Autodesk Inventor part; units mm, degrees
ref_plane "Work Plane1" through (0, 0, 110) normal (0, 0, 1) x (1, 0, 0)
ref_plane "Work Plane2" through (-77.5, 605, 280) normal (0, 1, 0) x (1, 0, 0)
ref_plane "Work Plane4" through (0, 0, 110) normal (0, 0, 1) x (1, 0, 0)
sketch "Sketch1" plane through (0, 0, 0) normal (0, 0, 1) x (1, 0, 0)
  line L0 (0, 450) -> (0, 610) construction
  line L1 (-77.5, 610) -> (-77.5, 443.2762)
  line L2 (77.5, 610) -> (77.5, 443.2762)
  arc A0 (77.5, 443.2762) -> (-77.5, 443.2762) centre (0, 0) ccw
  line L3 (-77.5, 610) -> (-77.5, 625)
  line L4 (-77.5, 625) -> (77.5, 625)
  line L5 (77.5, 625) -> (77.5, 610)
  dimension "d7" = 15
extrude "Extrusion1" add sketch "Sketch1" along normal blind 220
sketch "Sketch2" plane through (0, 0, 220) normal (0, 0, 1) x (1, 0, 0)
  arc A0 (77.5, 443.2762) -> (-77.5, 443.2762) centre (0, 0) ccw
  line L0 (77.5, 443.2762) -> (77.5, 625)
  line L1 (77.5, 458.4962) -> (77.5, 625)
  line L2 (77.5, 625) -> (-77.5, 625)
  line L3 (-77.5, 625) -> (-77.5, 458.4962)
  arc A1 (77.5, 458.4962) -> (-77.5012, 458.496) centre (0, 0) ccw
  dimension "d12" = 465
extrude "Extrusion2" add sketch "Sketch2" along normal blind 10
sketch "Sketch3" plane through (0, 0, 230) normal (0, 0, 1) x (1, 0, 0)
  arc A0 (77.5, 443.2762) -> (-77.5, 443.2762) centre (0, 0) ccw
  arc A1 (77.5, 443.2762) -> (-77.5, 443.2762) centre (0, 0) ccw
  line L0 (-77.5, 625) -> (-77.5, 443.2762)
  line L1 (-77.5, 443.2762) -> (-77.5, 625)
  line L2 (-77.5, 625) -> (77.5, 625)
  line L3 (77.5, 625) -> (77.5, 443.2762)
extrude "Extrusion3" add sketch "Sketch3" along normal blind 50
ref_plane "Work Plane1" through (0, 0, 110) normal (0, 0, 1) x (1, 0, 0)
mirror "Mirror1" about plane through (0, 0, 110) normal (0, 0, 1) of "Extrusion2", "Extrusion3"
ref_plane "Work Plane2" through (-77.5, 605, 280) normal (0, 1, 0) x (1, 0, 0)
sketch "Sketch4" plane through (-77.5, 605, 280) normal (0, 1, 0) x (1, 0, 0)
  line L0 (5, 15) -> (5, 325)
  line L1 (150, 15) -> (150, 325)
  line L2 (155, 340) -> (155, 0)
  line L3 (150, 15) -> (5, 15)
  line L4 (150, 325) -> (5, 325)
  point P0 (77.5, 280)
extrude "Extrusion4" cut sketch "Sketch4" against normal up to next
sketch "Sketch5" plane through (77.5, 443.2762, 220) normal (1, 0, 0) x (0, 0, -1)
  line L0 (280, 181.7238) -> (-60, 181.7238)
  line L1 (-60, 181.7238) -> (280, 181.7238)
  line L2 (-10, 0) -> (-60, 0)
  line L3 (-60, 0) -> (-60, 181.7238)
  line L4 (230, 0) -> (280, 0)
  line L5 (280, 181.7238) -> (280, 0)
  line L6 (280, 0) -> (280, 181.7238)
  line L7 (230, 0) -> (280, 0)
  line L8 (220, 15.22) -> (230, 15.22)
  line L9 (230, 0) -> (230, 15.22)
  line L10 (230, 15.22) -> (220, 15.22)
  line L11 (220, 15.22) -> (220, 0)
  line L12 (0, 16.0372) -> (0, 15.22)
  line L13 (0, 0) -> (0, 15.22)
  line L14 (0, 15.22) -> (-10, 15.22)
  line L15 (0, 15.22) -> (-10, 15.22)
  line L16 (-10, 15.22) -> (-10, 0)
  line L17 (-60, 0) -> (-10, 0)
  line L18 (0, 0) -> (220, 0)
  point P0 (220, -443.2762)
extrude "Extrusion5" add sketch "Sketch5" along normal blind 10
mirror "Mirror2" about plane through (0, 0, 0) normal (1, 0, 0) of "Extrusion5"
ref_plane "Work Plane4" through (0, 0, 110) normal (0, 0, 1) x (1, 0, 0)
sketch "Sketch7" plane through (0, 0, 110) normal (0, 0, 1) x (1, 0, 0)
  line L0 (87.5, 625) -> (87.5, 443.2762)
  arc A0 (-87.5, 625) -> (87.5, 625) centre (0, 0) ccw
  arc A1 (-87.5, 517.657) -> (87.5, 517.657) centre (0, 0) ccw
  line L1 (87.5, 517.657) -> (87.5, 625)
  line L2 (-87.5, 625) -> (-87.5, 517.657)
  dimension "d20" = 1050
extrude "Extrusion6" add sketch "Sketch7" along normal mid plane 100
sketch "Sketch8" plane through (0, 0, 160) normal (0, 0, 1) x (1, 0, 0)
  line L0 (0, 0) -> (-251.6368, -373.0669) construction
  line L1 (0, 0) -> (0, -450) construction
  line L2 (0, 0) -> (251.6368, -373.0669) construction
  line L3 (0, 0) -> (0, -450) construction
  line L4 (257.2287, -381.3573) -> (293.5763, -435.2447)
  arc A0 (-87.5, 517.657) -> (87.5, 517.657) centre (0, 0) ccw
  line L5 (-257.2287, -381.3573) -> (-293.5763, -435.2447)
  arc A1 (-293.5763, -435.2447) -> (293.5763, -435.2447) centre (0, 0) ccw
  arc A2 (0, -460) -> (257.2287, -381.3573) centre (0, 0) ccw
  arc A3 (-257.2287, -381.3573) -> (0, -460) centre (0, 0) ccw
  dimension "d24" = 34
  dimension "d25" = 34
  dimension "d28" = 450
  dimension "d29" = 460
extrude "Extrusion7" add sketch "Sketch8" against normal blind 100
sketch "Sketch9" plane through (0, 0, 110) normal (0, 0, 1) x (1, 0, 0)
  arc A0 (293.5763, -435.2447) -> (87.5, 517.657) centre (0, 0) ccw
  arc A1 (507.1111, -135.88) -> (507.1111, 135.88) centre (0, 0) ccw
  line L0 (0, 0) -> (507.1111, 135.88) construction
  line L1 (0, 0) -> (525, 0) construction
  line L2 (0, 0) -> (507.1111, -135.88) construction
  arc A2 (434.6666, -116.4686) -> (434.6666, 116.4686) centre (0, 0) ccw
  line L3 (0, 0) -> (434.6666, 116.4686) construction
  line L4 (0, 0) -> (450, 0) construction
  line L5 (0, 0) -> (434.6666, -116.4686) construction
  line L6 (434.6666, 116.4686) -> (507.1111, 135.88)
  line L7 (507.1111, -135.88) -> (434.6666, -116.4686)
  dimension "d30" = 15
  dimension "d31" = 30
  dimension "d32" = 450
  dimension "d33" = 15
  dimension "d34" = 30
extrude "Extrusion8" add sketch "Sketch9" along normal mid plane 220
sketch "Sketch10" plane through (0, 0, 220) normal (0, 0, 1) x (1, 0, 0)
  line L0 (507.1111, 135.88) -> (434.6666, 116.4686)
  arc A0 (449.1555, -120.3509) -> (449.1555, 120.3509) centre (0, 0) ccw
  arc A1 (507.1111, -135.88) -> (507.1111, 135.88) centre (0, 0) ccw
  arc A2 (507.1111, -135.88) -> (507.1111, 135.88) centre (0, 0) ccw
  line L1 (449.1555, 120.3509) -> (507.1111, 135.88)
  line L2 (507.1111, -135.88) -> (449.1555, -120.3509)
  dimension "d37" = 465
extrude "Extrusion9" add sketch "Sketch10" along normal blind 10
sketch "Sketch11" plane through (0, 0, 230) normal (0, 0, 1) x (1, 0, 0)
  arc A0 (434.6666, -116.4686) -> (434.6666, 116.4686) centre (0, 0) ccw
  line L0 (434.6666, 116.4686) -> (507.1111, 135.88)
  arc A1 (434.6666, -116.4686) -> (434.6666, 116.4686) centre (0, 0) ccw
  arc A2 (507.1111, -135.88) -> (507.1111, 135.88) centre (0, 0) ccw
  arc A3 (507.1111, -135.88) -> (507.1111, 135.88) centre (0, 0) ccw
  line L1 (507.1111, 135.88) -> (434.6666, 116.4686)
  line L2 (507.1111, -135.88) -> (434.6666, -116.4686)
  line L3 (507.1111, -135.88) -> (434.6666, -116.4686)
extrude "Extrusion10" add sketch "Sketch11" along normal blind 30
mirror "Mirror3" about plane through (0, 0, 110) normal (0, 0, 1) of "Extrusion9", "Extrusion10"
mirror "Mirror4" about plane through (0, 0, 0) normal (1, 0, 0) of "Extrusion8", "Extrusion9", "Extrusion10", "Mirror3"
ref_plane "Work Plane3" through (0, 0, 0) normal (1, 0, 0) x (0, 1, 0)
properties part number "source holder"
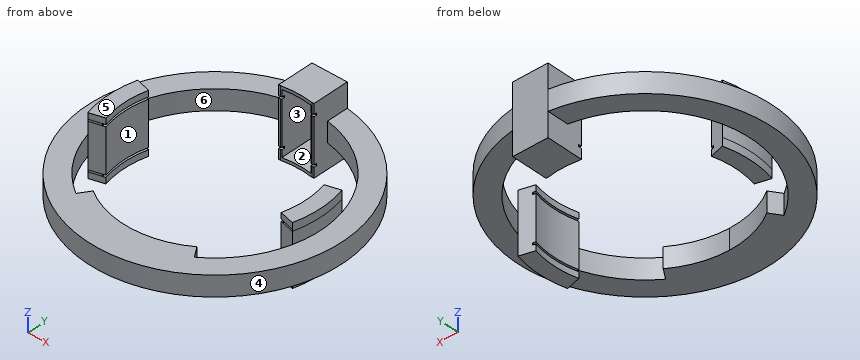
Input: part model. Units: mm. Frame: model coordinates. Face numbers are marked on the shaded views. A direction names the side the tool comes from. Give positions to 0.01 mm unless a question says otherwise; leave off trailing zeros. Loops run counter-clockwise (first coordinate to the right, second up) from the corner with the lowest first, then second, coordinate; pieces in that order, holes last. Notation, with made-up numbers: (-36, 69) - (-10, 69) arc R11 cw to (-10, 76) - close; hole circle Ø7 at (32, 35). An arc over 180 degrees is marked (long way). Use CSV: the item, a comma, the result in double quotes. Start each with the question number.
Item 1: Line query: line 1 (Z direction, x = -2, y = 569.5); line 2 (X direction, y = 501.5, z = 44); line 3 (X direction, y = -399, z = 116). Output: solid intervals per line, ascending.
Item 2: Reachability of the marked faces 1, 2 and 3 from +Z, -Z, +X, -X, +Y, -Y: full face, straight path, thin tool, end or side. Return the list, or none.
Item 3: Section A-A on y = 485. Return loops of the section in (x, z).
Item 4: Section B-B on x = -192. Return loops of the section in (y, z).
Item 5: Section D-D on y = -174. Return loops of the section in (x, z).
Item 6: Mould query, pull axis X, two halves, no side actions, for the marked faces 4, 5 and 6. Classes: pulls with the +X half, pulls with the -X half, needs draft (parallel to the pull), parting line crosses it, or undercut.
Item 7: Contact query for flat-ended pins moving along their axis: P1, Ø11, axis at x = 82.5, z = -3.5, coming from the -Y side; P2, Ø5, axis at x = 501.5, y = 101, coming from the +Z side; P3, Ø9, axis at x = 457, y = 12.5, coming from the -Z side. Output: stop coordinate, or through.
Item 8: Section C-C on z = 115.5. Return loops of the section in (x, y).
Ans:
1,line 1,"z = -60 to -45, 265 to 280"
1,line 2,"x = -87.5 to -72.5, 72.5 to 87.5"
1,line 3,"x = -488.96 to -341.21, -269.13 to -228.91, 228.91 to 269.13, 341.21 to 488.96"
2,face 1,"+Z, -Z"
2,face 2,"-Y"
2,face 3,"none"
3,outline,"(-403.8, 60) - (-201, 60) - (-201, 160) - (-403.8, 160) - close; (-87.5, -60) - (87.5, -60) - (87.5, 280) - (-87.5, 280) - close; (201, 60) - (403.8, 60) - (403.8, 160) - (201, 160) - close; hole (-72.5, -45) - (72.5, -45) - (72.5, 265) - (-72.5, 265) - close"
4,outline,"(-601.18, 60) - (-418.01, 60) - (-418.01, 160) - (-601.18, 160) - close; (488.63, 60) - (601.18, 60) - (601.18, 160) - (488.63, 160) - close"
5,outline,"(-606.63, 60) - (-495.33, 60) - (-495.33, 160) - (-606.63, 160) - close; (495.33, 60) - (606.63, 60) - (606.63, 160) - (495.33, 160) - close"
6,face 4,"parting line crosses it"
6,face 5,"needs draft"
6,face 6,"undercut"
7,P1,"stops at y = 443.28"
7,P2,"stops at z = 260"
7,P3,"stops at z = -40"
8,outline,"(-87.5, 625) arc R631.1 ccw (long way) to (87.5, 625) - close; hole (-507.11, -135.88) arc R525 ccw to (-293.58, -435.24) - (-257.23, -381.36) arc R460 ccw to (0, -460) arc R460 ccw to (257.23, -381.36) - (293.58, -435.24) arc R525 ccw to (507.11, -135.88) - (434.67, -116.47) arc R450 ccw to (434.67, 116.47) - (507.11, 135.88) arc R525 ccw to (87.5, 517.66) - (87.5, 443.28) - (77.5, 443.28) arc R450 ccw to (72.5, 444.12) - (72.5, 605) - (-72.5, 605) - (-72.5, 444.12) arc R450 ccw to (-77.5, 443.28) - (-87.5, 443.28) - (-87.5, 517.66) arc R525 ccw to (-507.11, 135.88) - (-434.67, 116.47) arc R450 ccw to (-434.67, -116.47) - close"
